from build123d import *

# Parameters (mm, degrees)
SKETCH2_W           = 78.486
SKETCH2_H           = 7.62
SKETCH2_R           = 2.7305
BOSS_EXTRUDE1_DEPTH = 9.271
SKETCH3_R           = 1.7272
CUT_EXTRUDE1_DEPTH  = 7.62
FILLET1_R           = 0.762


with BuildPart() as part:
    # Sketch2 → Boss-Extrude1 (new body)
    with BuildSketch(Plane(origin=(0, 0, 0), x_dir=(1, 0, 0), z_dir=(0, 1, 0))):
        with Locations((39.243, 3.81)):
            Rectangle(SKETCH2_W, SKETCH2_H)
        with Locations(Location((6.223, 3.81, 0), (0, 0, 270))):
            Circle(SKETCH2_R, mode=Mode.SUBTRACT)
        with Locations(Location((72.263, 3.81, 0), (0, 0, 270))):
            Circle(SKETCH2_R, mode=Mode.SUBTRACT)
    extrude(amount=BOSS_EXTRUDE1_DEPTH)

    # Sketch3 → Cut-Extrude1 (cut)
    with BuildSketch(Plane.XY):
        with Locations((17.018, 4.6355)):
            Circle(SKETCH3_R)
        with Locations((61.468, 4.6355)):
            Circle(SKETCH3_R)
    extrude(amount=-CUT_EXTRUDE1_DEPTH, mode=Mode.SUBTRACT)

    # Fillet1
    fillet1_edges = [part.edges().sort_by_distance(p)[0] for p in [
        (78.486, 9.271, -3.81),
        (39.243, 9.271, -7.62),
        (0, 9.271, -3.81),
        (39.243, 0, -7.62),
        (78.486, 0, -3.81),
        (39.243, 0, 0),
        (0, 0, -3.81),
        (39.243, 9.271, 0),
        (0, 4.6355, -7.62),
        (78.486, 4.6355, -7.62),
        (78.486, 4.6355, 0),
        (0, 4.6355, 0),
    ]]
    fillet(fillet1_edges, radius=FILLET1_R)


solid = part.part
Can you work these out from the model? Positions are in its coordinate system, mm. Give positions to 0.01 mm unless a question says otherwise; leave off trailing zeros. Write each loop counter-clockwise with the first axis right and the second up, starting at its lowest first coordinate (ties: lowest second). Pieces come first, ordered by that corner, then holes. Notation, with made-up numbers: (62, 29) -> (107, 29) arc R31 ccw to (107, 66) -> close; hole circle Ø10 at (-5, 25). An arc over 180 degrees is marked (long way). Answer as a JSON object with one key per item and string values. Group by question number.
Item 1: Suppose I cut it at C-C (x = 17). Please give me the cut outline in (y, z).
Item 2: Suppose I cut it at B-B (y = 5.5). Please give me the cut outline in (x, z), plus the area to 3 significant figures.
Item 3: Please list where these lines run through material, in increasing order: line 1 (X direction, y = 2.75, z = -4); line 2 (X direction, y = 2, z = -3.81); line 3 (Z direction, x = 72.5, y = 7). Write a range as [from, to].
Item 4: Suppose I cut it at D-D (x = 61). Please give me the cut outline in (y, z).
Item 5: Suppose I cut it at A-A (z = -5.25). Please give me the cut outline in (x, y), plus the area to 3 significant figures.
Item 6: We'd pull the mould along Z, two halves only. Please class faces 1 (the face through (39, 5, -7.62)), 2 (the face through (59.742, 4.711, -3.757)), 3 (the face through (74.565, 4.571, -2.342)): +Z half, -Z half, draft (parallel to the pull), parting line (faces both ways), or undercut.
Findings:
{
 "1": {"outline": "(0, -6.86) arc R0.76 ccw to (0.76, -7.62) -> (2.91, -7.62) -> (2.91, 0) -> (0.76, 0) arc R0.76 ccw to (0, -0.76) -> close; (6.36, -7.62) -> (8.51, -7.62) arc R0.76 ccw to (9.27, -6.86) -> (9.27, -0.76) arc R0.76 ccw to (8.51, 0) -> (6.36, 0) -> close"},
 "2": {"outline": "(0, -6.86) arc R0.76 ccw to (0.76, -7.62) -> (15.52, -7.62) -> (15.52, 0) -> (0.76, 0) arc R0.76 ccw to (0, -0.76) -> close; (18.51, -7.62) -> (59.97, -7.62) -> (59.97, 0) -> (18.51, 0) -> close; (62.96, -7.62) -> (77.72, -7.62) arc R0.76 ccw to (78.49, -6.86) -> (78.49, -0.76) arc R0.76 ccw to (77.72, 0) -> (62.96, 0) -> close; hole circle Ø5.46 at (6.22, -3.81); hole circle Ø5.46 at (72.26, -3.81)", "area": "505 mm²"},
 "3": {"line 1": "x = [0, 3.5], [8.95, 69.54], [74.99, 78.49]", "line 2": "x = [0, 3.49], [8.95, 69.53], [74.99, 78.49]", "line 3": "z = [-7.62, -6.53], [-1.09, 0]"},
 "4": {"outline": "(0, -6.86) arc R0.76 ccw to (0.76, -7.62) -> (2.97, -7.62) -> (2.97, 0) -> (0.76, 0) arc R0.76 ccw to (0, -0.76) -> close; (6.3, -7.62) -> (8.51, -7.62) arc R0.76 ccw to (9.27, -6.86) -> (9.27, -0.76) arc R0.76 ccw to (8.51, 0) -> (6.3, 0) -> close"},
 "5": {"outline": "(0, 0.76) arc R0.76 ccw to (0.76, 0) -> (3.9, 0) -> (3.9, 9.27) -> (0.76, 9.27) arc R0.76 ccw to (0, 8.51) -> close; (8.54, 0) -> (69.94, 0) -> (69.94, 9.27) -> (8.54, 9.27) -> close; (74.58, 0) -> (77.72, 0) arc R0.76 ccw to (78.49, 0.76) -> (78.49, 8.51) arc R0.76 ccw to (77.72, 9.27) -> (74.58, 9.27) -> close; hole circle Ø3.45 at (17.02, 4.64); hole circle Ø3.45 at (61.47, 4.64)", "area": "622 mm²"},
 "6": {"face 1": "-Z half", "face 2": "draft", "face 3": "undercut"}
}
